Here's how the part is built. I have some questions about the finished solid (model axes, mm). Give positions to 0.01 mm unless a question says otherwise; leave off trailing zeros. Loops run counter-clockwise (first coordinate to the right, second up) from the corner with the lowest first, then second, coordinate; pieces in that order, holes last. Notation, with made-up numbers: (75, 0.5) - (122, 0.5) arc R29 ccw to (122, 39.5) - close; hole circle Ø6 at (73, 40.5). An arc over 180 degrees is marked (long way). Use one line per item in the form item = value.
from build123d import *

# Parameters (mm, degrees)
SKETCH1_W           = 304.8
SKETCH1_H           = 457.2
BOSS_EXTRUDE1_DEPTH = 2.54
BOSS_EXTRUDE2_DEPTH = 0.254


with BuildPart() as part:
    # Sketch1 → Boss-Extrude1 (new body)
    with BuildSketch(Plane.XY):
        with Locations((152.4, 228.6)):
            Rectangle(SKETCH1_W, SKETCH1_H)
    extrude(amount=BOSS_EXTRUDE1_DEPTH)

    # Sketch2 → Boss-Extrude2 (add)
    with BuildSketch(Plane.XY.offset(2.54)):
        Polygon((76.582640735, 188.599807008), (116.844272896, 188.599807008), (116.844272896, 214.220845657), (101.157922704, 214.220845657), (101.157922704, 282.717908165), (140.896676525, 188.599807008), (179.13215512, 282.717908165), (179.13215512, 214.220845657), (167.067091951, 214.220845657), (167.067091951, 188.599807008), (232.753082879, 188.599807008), (232.753082879, 214.220845657), (222.900184239, 214.220845657), (222.900184239, 282.717908165), (232.753082879, 282.717908165), (232.753082879, 309.27172291), (222.900184239, 309.27172291), (162.34351535, 309.27172291), (140.896676525, 256.479504264), (118.606628652, 309.27172291), (59.196762562, 309.27172291), (45.234909284, 309.27172291), (45.234909284, 282.717908165), (59.196762562, 282.717908165), (59.196762562, 214.220845657), (45.234909284, 214.220845657), (45.234909284, 188.599807008), align=None)
    extrude(amount=BOSS_EXTRUDE2_DEPTH)


solid = part.part
(1) For P1, Ø1, axis at x = 236, y = 68.5, coming from the +Z side, with a flat end and sliding along its axis, tell me the tip position at first contact or that it passes through.
Geometry says:
P1 = 2.54
(2) If we section it at C-C (x = 25): List the corners of the cut face in (y, z) for me.
Geometry says:
outline = (0, 0) - (457.2, 0) - (457.2, 2.54) - (0, 2.54) - close
(3) If I drill on probe 1 along Z at (x, y) = (168, 113.5), over which ranges is the centre line in solid material (lowest first)?
Geometry says:
probe_1 = 0 to 2.54
(4) If we section it at B-B (y = 193): List the corners of the cut face in (x, z) for me.
Geometry says:
outline = (0, 0) - (304.8, 0) - (304.8, 2.54) - (232.75, 2.54) - (232.75, 2.79) - (167.07, 2.79) - (167.07, 2.54) - (142.68, 2.54) - (142.68, 2.79) - (139.04, 2.79) - (139.04, 2.54) - (116.84, 2.54) - (116.84, 2.79) - (45.23, 2.79) - (45.23, 2.54) - (0, 2.54) - close
(5) If we section it at D-D (y = 295): List the corners of the cut face in (x, z) for me.
Geometry says:
outline = (0, 0) - (304.8, 0) - (304.8, 2.54) - (232.75, 2.54) - (232.75, 2.79) - (156.55, 2.79) - (156.55, 2.54) - (124.63, 2.54) - (124.63, 2.79) - (45.23, 2.79) - (45.23, 2.54) - (0, 2.54) - close
(6) If we section it at A-A (x = 187.5): List the corners of the cut face in (y, z) for me, plus the area to 3 significant figures.
Geometry says:
outline = (0, 0) - (457.2, 0) - (457.2, 2.54) - (309.27, 2.54) - (309.27, 2.79) - (188.6, 2.79) - (188.6, 2.54) - (0, 2.54) - close
area = 1,190 mm²
